Geometry check sheet. Reference: drawing and pictorial views, mm from the part's lowest x, y, z. Round coordinates to 2 decimals unless told otherwise and drop trailing zeros. Order: outer loops, then holes, each group sorted by start corner. A loop starts at its lowest first (then second) coordinate and runs counter-clockwise, first axis right, second up. Notation, with made-up numbers: (13.5, 83.25) -> (19.5, 83.25) arc R19 cw to (19.5, 110.25) -> close; hole circle Ø6 at (-11, 78). An arc over 180 degrees is marked (long way). Put each result on its own line as item: value.
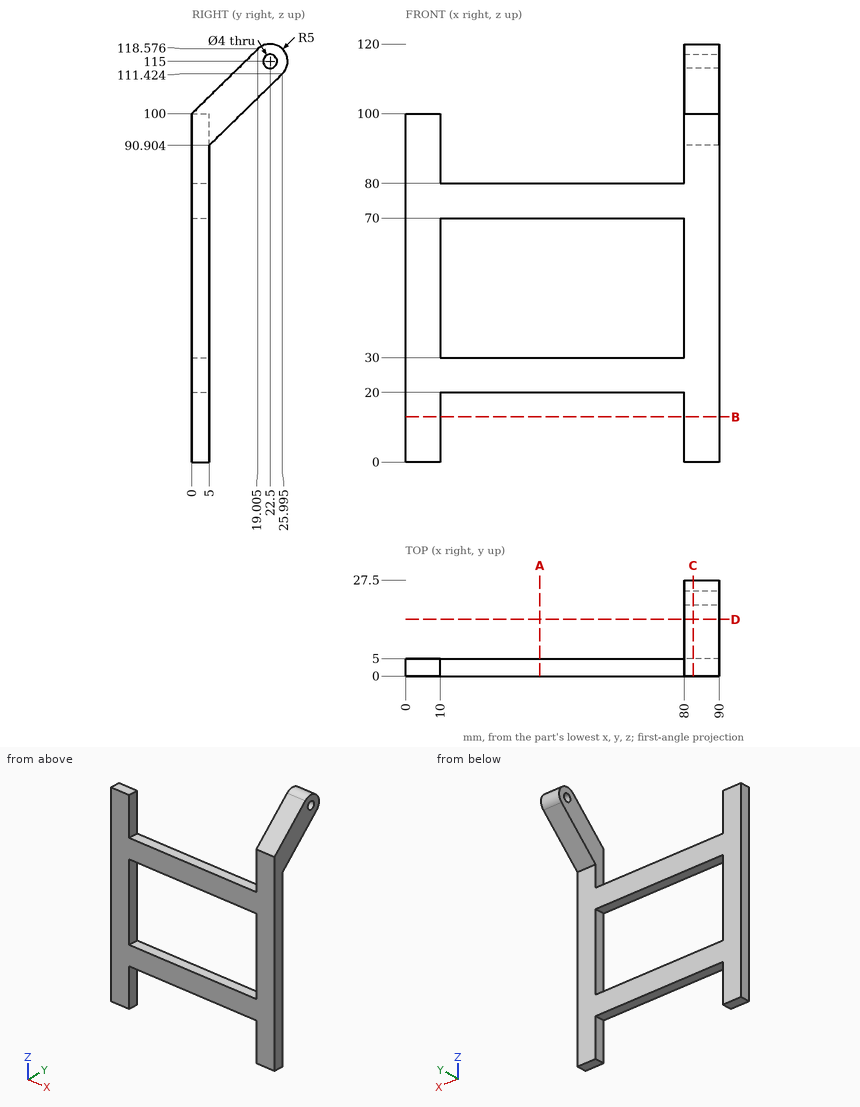
Item 1: Sectioned sample at D-D, the plane y = 16.25. Record the boundary of the cut face in (x, z), then the cut area to 3 significant figures.
Geometry check:
outline: (80, 101.9) -> (90, 101.9) -> (90, 115.88) -> (80, 115.88) -> close
area: 140 mm2
Item 2: Sectioned sample at B-B, the plane z = 13. Record the boundary of the cut face in (x, y).
Geometry check:
outline: (0, 0) -> (10, 0) -> (10, 5) -> (0, 5) -> close; (80, 0) -> (90, 0) -> (90, 5) -> (80, 5) -> close
Item 3: Sectioned sample at C-C, the plane x = 82.5. Record the boundary of the cut face in (y, z) (1 decimal).
Geometry check:
outline: (0, 0) -> (5, 0) -> (5, 90.9) -> (26, 111.4) arc R5 ccw to (19, 118.6) -> (0, 100) -> close; hole circle Ø4 at (22.5, 115)
Item 4: Depth check by flat-ended pin: pin 1 Ø6 at (y, z) = (9.5, 96) entering from -X; pin 2 Ø2.5 at (x, y) = (30, 2) entering from +Z; pin 3 Ø2.5 at (x, y) = (48.5, 2.5) entering from -Z. Enter the tip coordinate at first touch or a pass-through.
Geometry check:
pin 1: x = 80
pin 2: z = 80
pin 3: z = 20
Item 5: Sectioned sample at A-A, the plane x = 38.5. Record the boundary of the cut face in (y, z), then the cut area to 3 significant figures.
Geometry check:
outline: (0, 20) -> (5, 20) -> (5, 30) -> (0, 30) -> close; (0, 70) -> (5, 70) -> (5, 80) -> (0, 80) -> close
area: 100 mm2
Item 6: Material ranges on line 1 along Z through (x, y) = (78.5, 1.5); line 2 along Y through (x, z) = (82, 115) (1 decimal); line 3 along X through (y, z) = (13.5, 106.5), recorded low to high.
Geometry check:
line 1: 20 to 30, 70 to 80
line 2: 15.3 to 20.5, 24.5 to 27.5
line 3: 80 to 90
